Design review of the part shown in the three views and the two pictorial views. Dimensions are in mm from the part's minimum x, y and z. A direction names the side the tool comes from. Give positions to 0.01 mm unless a question says otherwise; leave off trailing zeros. Loops run counter-clockwise (first coordinate to the right, second up) from the corner with the lowest first, then second, coordinate; pieces in that order, holes last. Notation, with made-up numbers: (11.25, 8.25) -> (19.25, 8.25) arc R36 ccw to (19.25, 43.25) -> close; hole circle Ø2 at (48, -4). An arc over 180 degrees is marked (long way). Use CSV: the item, a comma, the result in double quotes. Start each with the question number.
Item 1: We need section C-C (y = 6.75). State the section outline as (x, z) points.
Item 2: For the marked faces 1, 2 and 3, list the 3-axis set-ups (+Z, -Z, +X, -X, +Y, -Y) from which the entire face can be reached by the end or side of a thin tool; tool diameter is ignored.
Item 3: We need section A-A (x = 1.5). State the section outline as (y, z) points.
Item 4: Wall thickness on line 1 along Y through (x, z) = (2.7, 1.45); line 2 along X through (y, z) = (6, 1.5): over which ranges is each line inside the solid? List them lowest first. Write a range as from..to.
Item 5: We need section B-B (z = 2.05). State the section outline as (x, y) points, plus the area to 3 significant figures.
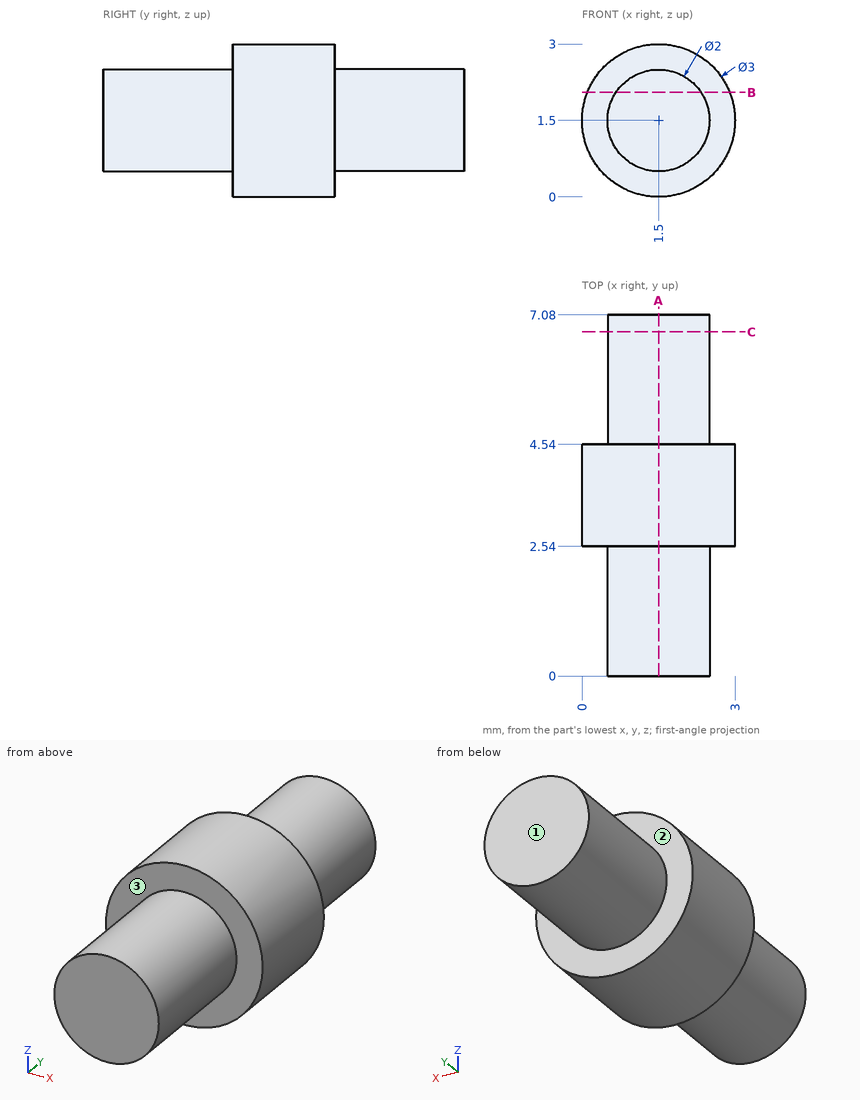
Results found:
1,outline,"circle Ø2 at (1.5, 1.5)"
2,face 1,"+Z, -Z, +X, -X, +Y"
2,face 2,"+Y"
2,face 3,"-Y"
3,outline,"(0, 0.5) -> (2.54, 0.5) -> (2.54, 0) -> (4.54, 0) -> (4.54, 0.5) -> (7.08, 0.5) -> (7.08, 2.5) -> (4.54, 2.5) -> (4.54, 3) -> (2.54, 3) -> (2.54, 2.5) -> (0, 2.5) -> close"
4,line 1,"2.54..4.54"
4,line 2,"0.5..2.5"
5,outline,"(0.1, 2.54) -> (0.66, 2.54) -> (0.66, 0) -> (2.34, 0) -> (2.34, 2.54) -> (2.9, 2.54) -> (2.9, 4.54) -> (2.34, 4.54) -> (2.34, 7.08) -> (0.66, 7.08) -> (0.66, 4.54) -> (0.1, 4.54) -> close"
5,area,"14.1 mm²"
